```python
from build123d import *

# Parameters (mm, degrees)
SKETCH2_R           = 137.922
SKETCH2_R_2         = 122.682
BOSS_EXTRUDE2_DEPTH = 1.5875
SKETCH3_W           = 290.977734258
SKETCH3_H           = 504.828840158
CUT_EXTRUDE1_DEPTH  = 205.235122161
BOSS_EXTRUDE3_DEPTH = 1.5875
FILLET2_R           = 6.35
FILLET3_R           = 12.7
SKETCH5_W           = 3.302
SKETCH5_H           = 10.16
SKETCH5_H_2         = 10.320651629
CUT_EXTRUDE2_DEPTH  = 219.975089365


with BuildPart() as part:
    # Sketch2 → Boss-Extrude2 (new, symmetric)
    with BuildSketch(Plane(origin=(248.273568551, -245.01347209, 0), x_dir=(0, -1, 0), z_dir=(0, 0, -1))):
        with Locations(Location((-257.71347209, 248.273568551, 0), (0, 0, 180))):
            Circle(SKETCH2_R)
        with Locations(Location((-257.71347209, 248.273568551, 0), (0, 0, 180))):
            Circle(SKETCH2_R_2, mode=Mode.SUBTRACT)
    extrude(amount=BOSS_EXTRUDE2_DEPTH, both=True)

    # Sketch3 → Cut-Extrude1 (cut, through all)
    with BuildSketch(Plane(origin=(0, 0, 0), x_dir=(0, 0, -1), z_dir=(1, 0, 0))):
        with Locations((4.206907001, 10.947122083)):
            Rectangle(SKETCH3_W, SKETCH3_H)
    extrude(amount=CUT_EXTRUDE1_DEPTH, mode=Mode.SUBTRACT)

    # Sketch4 → Boss-Extrude3 (add, symmetric)
    with BuildSketch(Plane.XY):
        with BuildLine():
            Line((-158.91199531, -30.452559211), (-104.007060596, -85.469026207))
            ThreePointArc((-104.007060596, -85.469026207), (-101.940396796, -83.943553525), (-99.869204781, -82.424234664))
            ThreePointArc((-99.869204781, -82.424234664), (-121.945025923, -51.735150773), (-134.859098706, -16.205044198))
            Line((-134.859098706, -16.205044198), (-158.91199531, -30.452559211))
        make_face()
    extrude(amount=BOSS_EXTRUDE3_DEPTH, both=True)

    # Fillet2
    # the kernel refuses this fillet: 6.35 mm, written as the material it adds along each edge
    with BuildSketch(Plane(origin=(-99.869204781, -82.424234664, 1.5875), x_dir=(0.7036137196097393, -0.7105826718805821, 0), z_dir=(0, 0, -1))) as fillet2_piece_1:
        with BuildLine():
            CenterArc((5.474610705, 6.348804924), FILLET2_R, 191.50159108, 77.386791497)
            Line((-0.747876011, 5.082645744), (-0.872325745, 5.057322561))
            ThreePointArc((-0.872325745, 5.057322561), (-0.503364548, 2.522278655), (-0.12559154, -0.018861738))
            Line((-0.12559154, -0.018861738), (0.002463821, -0.126976098))
            ThreePointArc((0.002463821, -0.126976098), (2.675709823, -0.101042949), (5.348955824, -0.126976098))
            Line((5.348955824, -0.126976098), (5.351419645, 0))
        make_face()
    extrude(amount=3.175)

    # Fillet3
    fillet3_edges = [part.edges().sort_by_distance(p)[0] for p in [
        (-134.859098706, -16.205044198, 0),
    ]]
    fillet(fillet3_edges, radius=FILLET3_R)

    # Sketch5 → Cut-Extrude2 (cut, through all)
    with BuildSketch(Plane(origin=(0, 0, -1.5875), x_dir=(-1, 0, 0), z_dir=(0, 0, -1))):
        with Locations((1.651, 146.812)):
            Rectangle(SKETCH5_W, SKETCH5_H)
        Polygon((109.043255392, 81.788598611), (110.732355392, 78.862991592), (120.034009933, 84.233304346), (118.344909933, 87.158911365), align=None)
        with Locations((1.651, -121.492325815)):
            Rectangle(SKETCH5_W, SKETCH5_H_2)
        Polygon((112.665009205, -50.115536994), (114.354109205, -47.189929975), (136.351154461, -59.889929975), (134.662054461, -62.815536994), align=None)
    extrude(amount=-CUT_EXTRUDE2_DEPTH, mode=Mode.SUBTRACT)


solid = part.part
```
Here's how the part is built. I have some questions about the finished solid (model axes, mm). A direction names the side the tool comes from. Round coordinates to 2 decimals unless told otherwise and drop trailing zeros. Loops run counter-clockwise (first coordinate to the right, second up) from the corner with the lowest first, then second, coordinate; pieces in that order, holes last.
1. Suppose I cut it at A-A, the plane x = -27. Please give me the cut outline in (y, z), and give its area (3 significant figures).
Answers:
outline: (-122.55, -1.59) - (-106.97, -1.59) - (-106.97, 1.59) - (-122.55, 1.59) - close; (132.37, -1.59) - (147.95, -1.59) - (147.95, 1.59) - (132.37, 1.59) - close
area: 98.9 mm2
2. Suppose I cut it at C-C, the plane y = 12.7. Please give me the cut outline in (x, z), and give its area (3 significant figures).
Answers:
outline: (-137.92, -1.59) - (-122.68, -1.59) - (-122.68, 1.59) - (-137.92, 1.59) - close
area: 48.4 mm2
3. For faces 1 (the face through (-52.72, -114.75, -0.02)), 2 (the face through (-123.07, -52.22, -0.02)), which set-ups out of +Z, -Z, +X, -X, +Y, -Y let a thin tool reach every point of the face, with its end or its side?
Answers:
face 1: +Z, -Z, -X, -Y
face 2: +Z, -Z
4. If I drill on probe 1 along Y at (x, z) = (-94.5, 0.05); probe 2 along Y at (x, z) = (-124, 0.6); probe 3 along X at (y, z) = (-51.5, -0.7), over which ranges is the centre line in solid material (lowest first)?
Answers:
probe 1: y = -87.76 to -65.53, 90.93 to 113.16
probe 2: y = -65.44 to -56.66, -52.76 to 73.09
probe 3: x = -137.91 to -121.82, -115.06 to -104.54
5. Will these pins go through, and if not, where does the flat tip stop? pin 1 (1.6 mm diameter, centred on y = -119, z = 0, fed in from +X); pin 2 (1 mm diameter, centred on y = -47.5, z = -0.5, fed in from -X).
Answers:
pin 1: stops at x = -3.3
pin 2: stops at x = -142.4
6. Thinking about a two-plate mould opening in X: for faces 3 (the face through (-137.507, -15.322, -0.022)), 4 (the face through (-121.23, -55.06, -0.02)), 5 (the face through (-125, 3, -1.588)), which applies, released by +X, released by -X, zero draft, split by the parting line, or undercut?
Answers:
face 3: released by -X
face 4: undercut
face 5: zero draft
7. Suppose I cut it at D-D, the plane x = -53.5. Please give me the cut outline in (y, z), and give its area (3 significant figures).
Answers:
outline: (-114.42, -1.59) - (-97.7, -1.59) - (-97.7, 1.59) - (-114.42, 1.59) - close; (123.1, -1.59) - (139.82, -1.59) - (139.82, 1.59) - (123.1, 1.59) - close
area: 106 mm2
